```python
from build123d import *

# Parameters (mm, degrees)
F0_R     = 325
F1_DEPTH = 75
F2_R     = 300
F3_DEPTH = 55
F4_R     = 20
F6_DEPTH = 25


with BuildPart() as f1:
    # F0 (on Top) → F1 (new body)
    with BuildSketch(Plane.XY):
        with Locations((0, 2.7766637504)):
            Circle(F0_R)
    extrude(amount=F1_DEPTH)

    # F2 (on face) → F3 (cut)
    with BuildSketch(Plane.XY.offset(75)):
        Circle(F2_R)
    extrude(amount=-F3_DEPTH, mode=Mode.SUBTRACT)

    # F4
    f4_edges = [f1.edges().sort_by_distance(p)[0] for p in [
        (-325, 2.776664, 0),
    ]]
    fillet(f4_edges, radius=F4_R)

    # F5 (on face) → F6 (cut)
    with BuildSketch(Plane.XY.offset(20)):
        with BuildLine():
            ThreePointArc((-3.9984777127, 72.3896551724), (0, 68.5), (3.9984777127, 72.3896551724))
            ThreePointArc((3.9984777127, 72.3896551724), (0, 72.5), (-3.9984777127, 72.3896551724))
        make_face()
        with BuildLine():
            ThreePointArc((-3.9984777127, 72.3896551724), (0, 72.5), (3.9984777127, 72.3896551724))
            ThreePointArc((3.9984777127, 72.3896551724), (3.9996194101, 72.4448223362), (4, 72.5))
            ThreePointArc((4, 72.5), (-0.0551776638, 76.4996194101), (-3.9984777127, 72.3896551724))
        make_face()
        with BuildLine():
            ThreePointArc((4, -72.5), (3.9996194101, -72.4448223362), (3.9984777127, -72.3896551724))
            ThreePointArc((3.9984777127, -72.3896551724), (0, -72.5), (-3.9984777127, -72.3896551724))
            ThreePointArc((-3.9984777127, -72.3896551724), (-0.0551776638, -76.4996194101), (4, -72.5))
        make_face()
        with BuildLine():
            ThreePointArc((-3.9984777127, -72.3896551724), (0, -72.5), (3.9984777127, -72.3896551724))
            ThreePointArc((3.9984777127, -72.3896551724), (0, -68.5), (-3.9984777127, -72.3896551724))
        make_face()
    extrude(amount=-F6_DEPTH, mode=Mode.SUBTRACT)


solid = f1.part
```
Verification items for the finished model (mm, model axes). A direction names the side the tool comes from. Give positions to 0.01 mm unless a question says otherwise; leave off trailing zeros. Write each loop counter-clockwise with the first axis right and the second up, starting at its lowest first coordinate (ties: lowest second). Pieces come first, ordered by that corner, then holes. Notation, with made-up numbers: (7.5, -31) - (29.5, -31) arc R29 cw to (29.5, 8) - close; hole circle Ø9 at (-11.75, 10.5). An arc over 180 degrees is marked (long way). Put each result on its own line as item: value.
Q1. Depth check by flat-ended pin: P1, Ø3, axis at x = 253, z = 34.5, coming from the +Y side; P2, Ø1, axis at x = 243.5, y = 104, coming from the +Z side; P3, Ø1.5, axis at y = -213.5, z = 23, coming from the -X side. Enter the tip coordinate at first touch or a pass-through.
Result:
P1: y = 208.62
P2: z = 20
P3: x = -243.26
Q2. Section check A-A on z = 44. Record the cut outline in (x, y).
Result:
outline: circle Ø650 at (0, 2.78); hole circle Ø600 at (0, 0)
Q3. Set-up check for faces 4 (the face through (71, 293, 75)), 5 (the face through (-39.054, 297.447, 47.885)): record each of +Z, -Z, +X, -X, +Y, -Y from which the full face is reachable in a straight line by a thin tool's end or side.
Result:
face 4: +Z, +X, -X, +Y, -Y
face 5: +Z
Q4. Scan lines: probe 1 along Y at (x, z) = (0, 46); probe 2 along X at (y, z) = (-71, 53.5); probe 3 along X at (y, z) = (110.5, 50). Record each from-to range of solid material in increasing order. Write a range as from..to.
Result:
probe 1: -322.22..-300, 300..327.78
probe 2: -316.52..-291.48, 291.48..316.52
probe 3: -306.63..-278.91, 278.91..306.63
Q5. Mould release check, pull along X, two halves, no side actions. Record for faces 1 (the face through (309.99, 100.4, 47.11)), 2 (the face through (-4, 7, 0)), 3 (the face through (-4, 4, 20)): released by +X, released by -X, zero draft, split by the parting line, or undercut.
Result:
face 1: split by the parting line
face 2: zero draft
face 3: undercut
